from build123d import *

# Parameters (mm, degrees)
SKETCH_1_W          = 90
SKETCH_1_H          = 48
EXTRUDE_1_DEPTH     = 40
CUT_EXTRUDE_1_DEPTH = 40
CUT_EXTRUDE_2_DEPTH = 49
CUT_EXTRUDE_3_DEPTH = 49
CUT_EXTRUDE_4_DEPTH = 33
SKETCH_6_W          = 8
SKETCH_6_H          = 40
CUT_EXTRUDE_5_DEPTH = 41
SKETCH_7_W          = 20
SKETCH_7_H          = 13.155555556
CUT_EXTRUDE_6_DEPTH = 5
SKETCH_8_W          = 28.2
SKETCH_8_H          = 28
EXTRUDE_2_DEPTH     = 7.5
SKETCH_9_R          = 2.25
EXTRUDE_3_DEPTH     = 4
SKETCH_10_R         = 1.2
CUT_EXTRUDE_7_DEPTH = 84
FILLET_1_R          = 5
FILLET_2_R          = 2.5
SKETCH_11_W         = 14.62039328
SKETCH_11_H         = 48
CUT_EXTRUDE_8_DEPTH = 10


with BuildPart() as part:
    # 스케치1 → 보스-돌출1 (new body)
    with BuildSketch(Plane(origin=(0, 0, 0), x_dir=(0, 0, -1), z_dir=(1, 0, 0))):
        with Locations((45, 24)):
            Rectangle(SKETCH_1_W, SKETCH_1_H)
    extrude(amount=EXTRUDE_1_DEPTH)

    # 스케치2 → 컷-돌출1 (cut)
    with BuildSketch(Plane(origin=(40, 0, 0), x_dir=(0, 0, -1), z_dir=(1, 0, 0))):
        Polygon((79, 44), (83, 44), (83, 38), (85.598076211, 36.5), (83, 35), (83, 33.5), (90, 33.5), (90, 14.5), (83, 14.5), (83, 13), (85.598076211, 11.5), (83, 10), (83, 4), (79, 4), align=None)
        Polygon((0, 38), (63.304035288, 48), (0, 48), align=None)
        Polygon((0, 10), (63.304035288, 0), (0, 0), align=None)
    extrude(amount=-CUT_EXTRUDE_1_DEPTH, mode=Mode.SUBTRACT)

    # 스케치3 → 컷-돌출2 (cut, through all)
    with BuildSketch(Plane(origin=(0, 48, 0), x_dir=(1, 0, 0), z_dir=(0, 1, 0))):
        Polygon((0, 67.846768337), (20, 79), (20, 90), (0, 90), align=None)
    extrude(amount=-CUT_EXTRUDE_2_DEPTH, mode=Mode.SUBTRACT)

    # 스케치4 → 컷-돌출3 (cut, through all)
    with BuildSketch(Plane(origin=(0, 48, 0), x_dir=(1, 0, 0), z_dir=(0, 1, 0))):
        Polygon((40, 63.304035288), (14.807552651, 0), (40, 0), align=None)
    extrude(amount=-CUT_EXTRUDE_3_DEPTH, mode=Mode.SUBTRACT)

    # 스케치5 → 컷-돌출4 (cut)
    with BuildSketch(Plane(origin=(40, 0, 0), x_dir=(0, 0, -1), z_dir=(1, 0, 0))):
        Polygon((4.2, 34.488888889), (63.304035288, 34.488888889), (63.304035288, 48), (0, 38), (0, 10), (63.304035288, 0), (63.304035288, 13.511111111), (4.2, 13.511111111), (4.2, 17.422222222), (63.304035288, 17.422222222), (63.304035288, 30.577777778), (4.2, 30.577777778), align=None)
    extrude(amount=-CUT_EXTRUDE_4_DEPTH, mode=Mode.SUBTRACT)

    # 스케치6 → 컷-돌출5 (cut, through all)
    with BuildSketch(Plane(origin=(40, 0, 0), x_dir=(0, 0, -1), z_dir=(1, 0, 0))):
        with Locations((72, 24)):
            Rectangle(SKETCH_6_W, SKETCH_6_H)
    extrude(amount=-CUT_EXTRUDE_5_DEPTH, mode=Mode.SUBTRACT)

    # 스케치7 → 컷-돌출6 (cut)
    with BuildSketch(Plane.XY.offset(-63.304035288)):
        with Locations((30, 24)):
            Rectangle(SKETCH_7_W, SKETCH_7_H)
    extrude(amount=-CUT_EXTRUDE_6_DEPTH, mode=Mode.SUBTRACT)

    # 스케치8 → 보스-돌출2 (add)
    with BuildSketch(Plane.ZY):
        with Locations((-14.1, 24)):
            Rectangle(SKETCH_8_W, SKETCH_8_H)
    extrude(amount=EXTRUDE_2_DEPTH)

    # 스케치9 → 보스-돌출3 (add)
    with BuildSketch(Plane(origin=(0, 0, -79), x_dir=(-1, 0, 0), z_dir=(0, 0, -1))):
        with Locations((-30, 24)):
            Circle(SKETCH_9_R)
    extrude(amount=EXTRUDE_3_DEPTH)

    # 스케치10 → 컷-돌출7 (cut, through all)
    with BuildSketch(Plane(origin=(0, 0, -83), x_dir=(-1, 0, 0), z_dir=(0, 0, -1))):
        with Locations((-30, 24)):
            Circle(SKETCH_10_R)
    extrude(amount=-CUT_EXTRUDE_7_DEPTH, mode=Mode.SUBTRACT)

    # 필렛1
    fillet_1_edges = [part.edges().sort_by_distance(p)[0] for p in [
        (16.47898289, 32.533333333, -4.2),
        (16.47898289, 15.466666667, -4.2),
        (-7.5, 24, -28.2),
        (30, 48, -90),
        (30, 0, -90),
    ]]
    fillet(fillet_1_edges, radius=FILLET_1_R)

    # 필렛2
    fillet_2_edges = [part.edges().sort_by_distance(p)[0] for p in [
        (30, 14.5, -90),
        (30, 33.5, -90),
    ]]
    fillet(fillet_2_edges, radius=FILLET_2_R)

    # 스케치11 → 컷-돌출8 (cut)
    with BuildSketch(Plane(origin=(0, 0, -68), x_dir=(-1, 0, 0), z_dir=(0, 0, -1))):
        with Locations((-7.31019664, 24)):
            Rectangle(SKETCH_11_W, SKETCH_11_H)
    extrude(amount=CUT_EXTRUDE_8_DEPTH, mode=Mode.SUBTRACT)


solid = part.part
Design review of the part built by this model. Coordinates are the model's own, in mm. A direction names the side the tool comes from. Round coordinates to 2 decimals unless told otherwise and drop trailing zeros. Write each loop counter-clockwise with the first axis right and the second up, starting at its lowest first coordinate (ties: lowest second). Pieces come first, ordered by that corner, then holes. Notation, with made-up numbers: (3.25, 15) - (26.25, 15) arc R15 ccw to (26.25, 28) - close; hole circle Ø3 at (46.5, 77.25). An arc over 180 degrees is marked (long way). Use a Markdown table: item, result. Add a question column.
1. We need section D-D (y = 41). State the section outline as (x, z) points, then the cut area to 3 significant figures.
2. Mouldability with a two-part tool opening along Y and no side actions: class faces 1 (the face through (-4, 38, -14)), 2 (the face through (10, 33, -4.2)), 3 (the face through (28.962, 22.004, -80.972)) as +Y half, -Y half, draft (parallel to the pull), parting line (faces both ways), or undercut.
3. For faces 4 (the face through (24, 7, -63.304)), 5 (the face through (30, 41, -83)), 6 (the face through (29, 23, -83)), 7 (the face through (14, 24, -63.304)), list the 3-axis set-ups (+Z, -Z, +X, -X, +Y, -Y) from which the entire face can be reached by the end or side of a thin tool; tool diameter is ignored.
4. Clearance check with flat-ended pins moving along their axes: pin 1 (4 mm diameter, centred on x = 11, y = 6, fed in from +Z); pin 2 (10 mm diameter, centred on x = 1, y = 34, fed in from +Z); pin 3 (8 mm diameter, centred on x = 3.5, y = 10, fed in from -Z); pin 4 (12 mm diameter, centred on x = 23.5, z = -28.5, fed in from +Y). State where each tip first meets the part, or that it passes through.
5. We need section A-A (y = 24). State the section outline as (x, z) points.
6. We need section B-B (x = 11.5). State the section outline as (y, z) points.
7. Wall thickness on probe 1 along Y at (x, z) = (30, -81); probe 2 along Y at (x, z) = (30.5, -44); probe 3 along Z at (x, y) = (27, 41): over which ranges is each line inside the solid? List them lowest first.
8. We need section C-C (z = -43). State the section outline as (x, y) points, then the cut area to 3 significant figures.
Output:
| question | item | result |
|---|---|---|
| 1 | outline | (0, -67.85) - (0.27, -68) - (40, -68) - (40, -63.3) - (7, -63.3) - (7, -18.99) - (0, -18.99) - close; (14.62, -76) - (20, -79) - (40, -79) - (40, -76) - close; (20, -90) - (40, -90) - (40, -83) - (20, -83) - close |
| 1 | area | 706 mm2 |
| 2 | face 1 | +Y half |
| 2 | face 2 | draft |
| 2 | face 3 | undercut |
| 3 | face 4 | +Z, +X, -Y |
| 3 | face 5 | +X, -X |
| 3 | face 6 | -Z, +X, -X |
| 3 | face 7 | +Z, +X |
| 4 | pin 1 | stops at z = -63.3 |
| 4 | pin 2 | stops at z = 0 |
| 4 | pin 3 | stops at z = -68 |
| 4 | pin 4 | stops at y = 34.49 |
| 5 | outline | (-7.5, -23.2) arc R5 ccw to (-2.5, -28.2) - (0, -28.2) - (0, -67.85) - (0.27, -68) - (20, -68) - (20, -63.3) - (7, -63.3) - (7, 0) - (-7.5, 0) - close; (14.62, -76) - (20, -79) - (27.75, -79) - (27.75, -83) - (28.8, -83) - (28.8, -76) - close; (31.2, -83) - (32.25, -83) - (32.25, -79) - (40, -79) - (40, -76) - (31.2, -76) - close |
| 6 | outline | (0, -68) - (48, -68) - (48, -63.3) - (34.49, -63.3) - (34.49, -4.2) - (30.58, -4.2) - (30.58, -63.3) - (17.42, -63.3) - (17.42, -4.2) - (13.51, -4.2) - (13.51, -63.3) - (0, -63.3) - close |
| 7 | probe 1 | y = 0 to 4, 21.75 to 22.8, 25.2 to 26.25, 44 to 48 |
| 7 | probe 2 | y = 13.51 to 17.42, 30.58 to 34.49 |
| 7 | probe 3 | z = -90 to -83, -79 to -76, -68 to -63.3 |
| 8 | outline | (0, 3.21) - (7, 3.21) - (7, 13.51) - (31.92, 13.51) - (31.92, 17.42) - (7, 17.42) - (7, 30.58) - (31.92, 30.58) - (31.92, 34.49) - (7, 34.49) - (7, 44.79) - (0, 44.79) - close |
| 8 | area | 486 mm2 |
